Autodesk Inventor part; units mm, degrees
ref_plane "YZ Plane" through (0, 0, 0) normal (1, 0, 0) x (0, 1, 0)
ref_plane "XZ Plane" through (0, 0, 0) normal (0, 1, 0) x (-1, 0, 0)
ref_plane "XY Plane" through (0, 0, 0) normal (0, 0, 1) x (1, 0, 0)
sketch "Sketch1" plane through (0, 0, 0) normal (0, 0, 1) x (1, 0, 0)
  line L0 (374.65, -215.9) -> (-374.65, -215.9)
  line L1 (-374.65, -215.9) -> (-374.65, 215.9)
  line L2 (-374.65, 215.9) -> (374.65, 215.9)
  line L3 (374.65, 215.9) -> (374.65, -215.9)
  line L4 (374.65, -215.9) -> (-374.65, 215.9) construction
  line L5 (-374.65, -215.9) -> (374.65, 215.9) construction
  line L6 (-374.65, -88.9) -> (374.65, -88.9) construction
  line L7 (-374.65, 215.9) -> (-76.2, -88.9)
  line L8 (374.65, 215.9) -> (76.2, -88.9)
  line L9 (-76.2, -88.9) -> (-76.2, -215.9)
  line L10 (76.2, -88.9) -> (76.2, -215.9)
  line L11 (-349.25, 189.9596) -> (-349.25, 215.9)
  line L12 (349.25, 215.9) -> (349.25, 189.9596)
  point P0 (0, 0)
  dimension "d0" = 749.3
  dimension "d1" = 431.8
  dimension "d5" = 152.4
  dimension "d6" = 76.2
  dimension "d7" = 127
  dimension "d8" = 25.4
  dimension "d9" = 25.4
extrude "Plate1" add sketch "Sketch1" along normal blind 3.048 contours L0 L9 L7 L11 L2 L12 L8 L10
equation "\"d2\" = Thickness"
equation "\"BendRadius\" = Thickness"
equation "\"BendReliefWidth\" = Thickness"
equation "\"BendReliefDepth\" = 0.5 * Thickness"
equation "\"CornerReliefSize\" = 4 * Thickness"
equation "\"MinimumRemnant\" = 2 * Thickness"
equation "\"TransitionRadius\" = BendRadius"
equation "\"JacobiRadiusSize\" = BendRadius"
equation "\"GapSize\" = Thickness"
properties part number "trough_backplate"
Build history of the part. All positions in model axes, mm. Round coordinates to 2 decimals unless told otherwise and drop trailing zeros. Order: outer loops, then holes, each group sorted by start corner. A loop starts at its lowest first (then second) coordinate and runs counter-clockwise, first axis right, second up. Notation, with made-up numbers: (-4.5, -4.75) - (16.5, -4.75) arc R7 ccw to (16.5, 4.25) - close; hole circle Ø11 at (38.25, 49.25). An arc over 180 degrees is marked (long way). Use a Markdown table: item, result.
1) Saw through at C-C on x = 152. Write the cut outline in (y, z), and give its area (3 significant figures).
Recorded:
| item | result |
|---|---|
| outline | (-11.49, 0) - (215.9, 0) - (215.9, 3.05) - (-11.49, 3.05) - close |
| area | 693 mm² |
2) Saw through at A-A on z = 1.4. Write the cut outline in (x, y).
Recorded:
| item | result |
|---|---|
| outline | (-349.25, 189.96) - (-76.2, -88.9) - (-76.2, -215.9) - (76.2, -215.9) - (76.2, -88.9) - (349.25, 189.96) - (349.25, 215.9) - (-349.25, 215.9) - close |
3) Flat gauge pin, fed straight in: pin 1 Ø1.5 at (y, z) = (-147, 2.5) entering from -X. Where does the tip first touch, or does it go through?
Recorded:
| item | result |
|---|---|
| pin 1 | stops at x = -76.2 |
4) Wall check: L1, parallel to X at y = -164, z = 2.4; L2, parallel to X at y = -86, z = 1.7; L3, parallel to Y at x = 110.5, z = 2.2. Give the ranges that are in metal, low to high.
Recorded:
| item | result |
|---|---|
| L1 | x = -76.2 to 76.2 |
| L2 | x = -79.04 to 79.04 |
| L3 | y = -53.87 to 215.9 |
5) Saw through at B-B on y = -153.5. Write the cut outline in (x, z), and give its area (3 significant figures).
Recorded:
| item | result |
|---|---|
| outline | (-76.2, 0) - (76.2, 0) - (76.2, 3.05) - (-76.2, 3.05) - close |
| area | 465 mm² |
